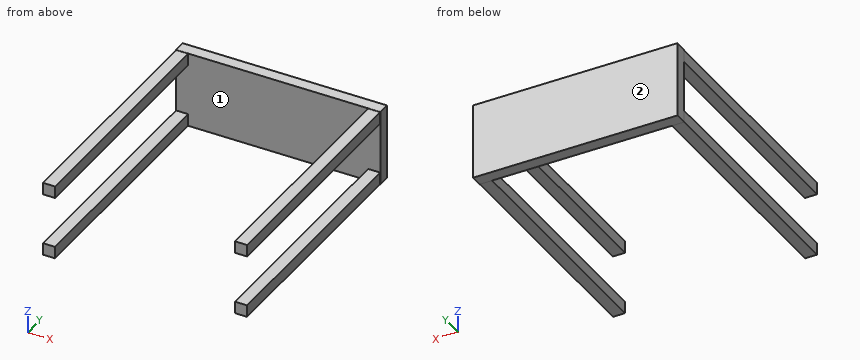
from build123d import *

# Parameters (mm, degrees)
F0_W     = 84.884792
F0_H     = 31.480454
F1_DEPTH = 5
F2_W     = 5
F2_H     = 5
F3_DEPTH = 105


with BuildPart() as f1:
    # F0 (on Front) → F1 (new body)
    with BuildSketch(Plane.XZ):
        Rectangle(F0_W, F0_H)
    extrude(amount=F1_DEPTH)

    # F2 (on Front) → F3 (join)
    with BuildSketch(Plane.XZ):
        with Locations((-39.864282, 13.145501)):
            Rectangle(F2_W, F2_H)
        with Locations((39.864282, 13.145501)):
            Rectangle(F2_W, F2_H)
        with Locations((39.864282, -13.145501)):
            Rectangle(F2_W, F2_H)
        with Locations((-39.864282, -13.145501)):
            Rectangle(F2_W, F2_H)
    extrude(amount=F3_DEPTH)


solid = f1.part
The listing builds one solid part. Answer for the finished solid, in the listing's coordinates (mm). Face numbers are marked on the shaded views. Give positions to 0.01 mm unless a question says otherwise; leave off trailing zeros. Write each loop counter-clockwise with the first axis right and the second up, starting at its lowest first coordinate (ties: lowest second). Pieces come first, ordered by that corner, then holes.
1) For a pull along X with two mould halves and no side action, classify the marked faces 1 and 2 as pulls with the +X half, pulls with the -X half, needs draft (parallel to the pull), parting line crosses it, or undercut.
2) Given P1, Ø5.5, axis at y = -31.5, z = 13, coming from the +X side; P2, Ø5.5, axis at x = -41, y = -62.5, coming from the +Z side; P3, Ø5.5, axis at y = -38, z = 14.5, coming from the -X side, each flat-ended and moving along its own axis, determine where each tip first touches the part or whether it passes through.
3) Section A-A (y = -74.5) is taken. Write down the section's boundary in (x, z), and give its area (3 significant figures).
4) Section B-B (z = -12.5) is taken. Write down the section's boundary in (x, y), and give its area (3 significant figures).
5) Section C-C (x = 15.5) is taken. Write down the section's boundary in (y, z).
6) Section D-D (z = -5) is taken. Write down the section's boundary in (x, y).
7) Find the intervals of material crossed by L1, parallel to Y at x = -33, z = -8.5, in increasing order.
Response:
1. face 1: undercut
1. face 2: needs draft
2. P1: stops at x = 42.36
2. P2: stops at z = 15.65
2. P3: stops at x = -42.36
3. outline: (-42.36, -15.65) - (-37.36, -15.65) - (-37.36, -10.65) - (-42.36, -10.65) - close; (-42.36, 10.65) - (-37.36, 10.65) - (-37.36, 15.65) - (-42.36, 15.65) - close; (37.36, -15.65) - (42.36, -15.65) - (42.36, -10.65) - (37.36, -10.65) - close; (37.36, 10.65) - (42.36, 10.65) - (42.36, 15.65) - (37.36, 15.65) - close
3. area: 100 mm2
4. outline: (-42.44, -5) - (-42.36, -5) - (-42.36, -105) - (-37.36, -105) - (-37.36, -5) - (37.36, -5) - (37.36, -105) - (42.36, -105) - (42.36, -5) - (42.44, -5) - (42.44, 0) - (-42.44, 0) - close
4. area: 1,420 mm2
5. outline: (-5, -15.74) - (0, -15.74) - (0, 15.74) - (-5, 15.74) - close
6. outline: (-42.44, -5) - (42.44, -5) - (42.44, 0) - (-42.44, 0) - close
7. L1: y = -5 to 0
